```python
from build123d import *

# Parameters (mm, degrees)
SKETCH_1_R        = 9.975
EXTRUDE_1_DEPTH   = 40
SKETCH_5_R        = 9.975
F_16MM_DEPTH      = 16
SKETCH_6_R        = 9.45
EXTRUDE_1_2_DEPTH = 1
SKETCH_7_R        = 9.975
EXTRUDE_4_DEPTH   = 44
SKETCH_8_R        = 9.45
EXTRUDE_2_DEPTH   = 1
SKETCH_9_R        = 9.975
EXTRUDE_6_DEPTH   = 2


with BuildPart() as part:
    # 草图1 → Extrude 1 (new body)
    with BuildSketch(Plane(origin=(0, 0, 0), x_dir=(1, 0, 0), z_dir=(0, 1, 0))):
        with Locations(Location((5.9, 0, 0), (0, 0, 270))):
            Circle(SKETCH_1_R)
    extrude(amount=EXTRUDE_1_DEPTH)

    # 草图5 → 16mm 铰链间距 (add)
    with BuildSketch(Plane(origin=(0, 40, 0), x_dir=(1, 0, 0), z_dir=(0, 1, 0))):
        with Locations(Location((5.9, 0, 0), (0, 0, 270))):
            Circle(SKETCH_5_R)
    extrude(amount=F_16MM_DEPTH)

    # 草图6 → Extrude 1 2 (add)
    with BuildSketch(Plane(origin=(0, 56, 0), x_dir=(1, 0, 0), z_dir=(0, 1, 0))):
        with Locations(Location((5.9, 0, 0), (0, 0, 270))):
            Circle(SKETCH_6_R)
    extrude(amount=EXTRUDE_1_2_DEPTH)

    # 草图7 → 凸台-拉伸4 (add)
    with BuildSketch(Plane(origin=(0, 57, 0), x_dir=(1, 0, 0), z_dir=(0, 1, 0))):
        with Locations(Location((5.9, 0, 0), (0, 0, 270))):
            Circle(SKETCH_7_R)
    extrude(amount=EXTRUDE_4_DEPTH)

    # 草图8 → 卡簧2 (add)
    with BuildSketch(Plane(origin=(0, 101, 0), x_dir=(1, 0, 0), z_dir=(0, 1, 0))):
        with Locations(Location((5.9, 0, 0), (0, 0, 270))):
            Circle(SKETCH_8_R)
    extrude(amount=EXTRUDE_2_DEPTH)

    # 草图9 → 凸台-拉伸6 (add)
    with BuildSketch(Plane(origin=(0, 102, 0), x_dir=(1, 0, 0), z_dir=(0, 1, 0))):
        with Locations(Location((5.9, 0, 0), (0, 0, 270))):
            Circle(SKETCH_9_R)
    extrude(amount=EXTRUDE_6_DEPTH)

    # 草图22 → M3 螺纹孔7 (revolve, cut)
    with BuildSketch(Plane(origin=(5.9, 8, 9.975), x_dir=(0, -1, 0), z_dir=(1, 0, 0))):
        Polygon((0, 0), (0, 8.251075774), (1.25, 7.5), (1.25, 0), align=None)
    hole_wizard_m3_7 = revolve(axis=Axis((5.9, 8, 16.325), (0, 0, -1)), mode=Mode.SUBTRACT)

    # 镜向1: M3 螺纹孔7 across plane
    add(hole_wizard_m3_7.mirror(Plane(origin=(0, 20, 0), x_dir=(0, 0, 1), z_dir=(0, -1, 0))), mode=Mode.SUBTRACT)


solid = part.part
```
Build history of the part. All positions in model axes, mm. A direction names the side the tool comes from. Give positions to 0.01 mm unless a question says otherwise; leave off trailing zeros. Loops run counter-clockwise (first coordinate to the right, second up) from the corner with the lowest first, then second, coordinate; pieces in that order, holes last.
1) Band-saw the part on B-B on x = 11.5. List the corners of the cut face in (y, z), then the cut area to 3 significant figures.
Values follow:
outline: (0, -8.25) - (56, -8.25) - (56, -7.61) - (57, -7.61) - (57, -8.25) - (101, -8.25) - (101, -7.61) - (102, -7.61) - (102, -8.25) - (104, -8.25) - (104, 8.25) - (102, 8.25) - (102, 7.61) - (101, 7.61) - (101, 8.25) - (57, 8.25) - (57, 7.61) - (56, 7.61) - (56, 8.25) - (0, 8.25) - close
area: 1,710 mm2
2) Band-saw the part on A-A on z = -6. List the corners of the cut face in (x, y), then the cut area to 3 significant figures.
Values follow:
outline: (-2.07, 0) - (13.87, 0) - (13.87, 56) - (13.2, 56) - (13.2, 57) - (13.87, 57) - (13.87, 101) - (13.2, 101) - (13.2, 102) - (13.87, 102) - (13.87, 104) - (-2.07, 104) - (-2.07, 102) - (-1.4, 102) - (-1.4, 101) - (-2.07, 101) - (-2.07, 57) - (-1.4, 57) - (-1.4, 56) - (-2.07, 56) - close
area: 1,650 mm2
3) Drop flat-ended pins along their axis: P1, Ø8, axis at y = 29.5, z = -6.5, coming from the -X side; P2, Ø5, axis at y = 68, z = 6, coming from the -X side; P3, Ø6, axis at x = 1, z = -1.5, coming from the -Y side; P4, Ø2, axis at x = 2.5, y = 56.5, coming from the +Z side. Give the stop position or say it passes through.
Values follow:
P1: stops at x = -3.76
P2: stops at x = -3.44
P3: stops at y = 0
P4: stops at z = 9.65
4) Band-saw the part on C-C on y = 47.5. List the corners of the cut face in (x, z) (3 decimals).
Values follow:
outline: circle Ø19.95 at (5.9, 0)
5) Probe line 1 along Y through (x, z) = (5.9, 6.5); line 2 along Y through (x, z) = (3.75, 9.25); line 3 along X through (y, z) = (36, -0.25). List the from-to ranges inside material, lowest first.
Values follow:
line 1: y = 0 to 6.75, 9.25 to 30.75, 33.25 to 104
line 2: y = 0 to 56, 57 to 101, 102 to 104
line 3: x = -4.07 to 15.87
6) Two-plate mould, pull along Y, no slides. Class faces 4 (the face through (-3, 101, 4)), 5 (the face through (-3.84, 102.99, -2.16)), 6 (the face through (6, 0, 0)), 7 (the face through (6, 104, 0)): released by +Y, released by -Y, zero draft, split by the parting line, or undercut.
Values follow:
face 4: undercut
face 5: zero draft
face 6: released by -Y
face 7: released by +Y
7) 3-axis set-ups, long thin cutter, end or side, ignore diameter. For faces 1 (the face through (8.739, 101.493, 9.014)), 2 (the face through (5.85, 9.25, 6.28)), 3 (the face through (-3.84, 27.61, -2.16)): which of +Z, -Z, +X, -X, +Y, -Y reach the whole face in a straight line?
Values follow:
face 1: none
face 2: +Z
face 3: +Y, -Y
8) Band-saw the part on D-D on z = 7. List the corners of the cut face in (x, y), then the cut area to 3 significant figures.
Values follow:
outline: (-1.21, 0) - (13.01, 0) - (13.01, 56) - (12.25, 56) - (12.25, 57) - (13.01, 57) - (13.01, 101) - (12.25, 101) - (12.25, 102) - (13.01, 102) - (13.01, 104) - (-1.21, 104) - (-1.21, 102) - (-0.45, 102) - (-0.45, 101) - (-1.21, 101) - (-1.21, 57) - (-0.45, 57) - (-0.45, 56) - (-1.21, 56) - close; hole circle Ø2.5 at (5.9, 8); hole circle Ø2.5 at (5.9, 32)
area: 1,470 mm2
